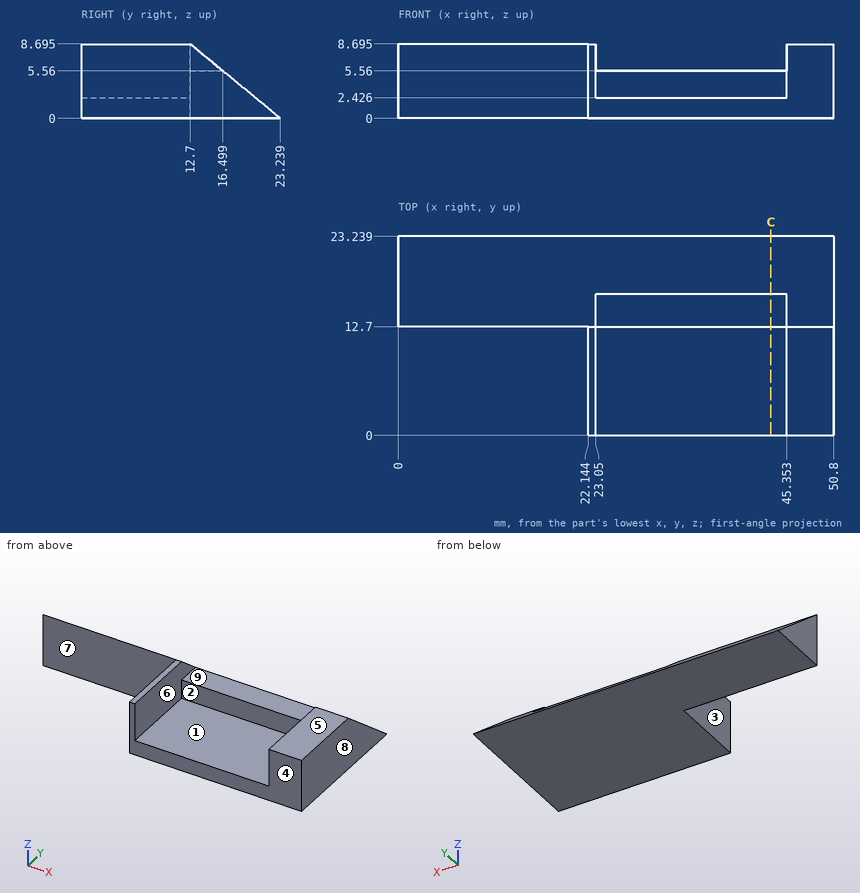
Verification items for this drawing (mm, ordinates from the low corner). A direction names the side the tool comes from. Coordinates: 2 decimals unless noted, no trailing zeros. Order: outer loops, then holes, each group sorted by start corner. A loop starts at its lowest first (then second) coordinate and runs counter-clockwise, first axis right, second up. Notation, with made-up numbers: (42, -38.75) -> (87, -38.75) arc R24 ccw to (87, -13.75) -> close; hole circle Ø4 at (80, 64). An arc over 180 degrees is marked (long way). Answer as CSV lines item,"result". Start each with the question number.
1) Release check for a two-part mould opening along X. For the marked faces 1, 2, 3 and 4 record: released by +X, released by -X, zero draft, split by the parting line, or undercut.
2) Gauge pin test, flat ends, axial feed: pin 1 Ø4 at (x, y) = (35.5, 6.5) entering from +Z; pin 2 Ø2.5 at (x, z) = (31.5, 4) entering from -Y; pin 3 Ø2.5 at (y, z) = (5.5, 4.5) entering from -X. Record the tip position at first contact, or that the pin passes through.
3) Material ranges on L1, parallel to Z at x = 35.5, y = 12.5; L2, parallel to X at y = 2.75, z = 0.5 (1 decimal); L3, parallel to Y at x = 11.5, z = 2.25, recorded low to high. Write a range as [from, to].
4) Set-up check for the marked faces 5, 6, 7, 8 and 9: record each of +Z, -Z, +X, -X, +Y, -Y from which the full face is reachable in a straight line by a thin tool's end or side.
5) Cross-section at C-C, the plane x = 43.5. Record the boundary of the cut face in (y, z).
Conclusion:
1,face 1,"undercut"
1,face 2,"undercut"
1,face 3,"released by -X"
1,face 4,"zero draft"
2,pin 1,"stops at z = 2.43"
2,pin 2,"stops at y = 12.7"
2,pin 3,"stops at x = 22.14"
3,L1,"z = [0, 2.43]"
3,L2,"x = [22.1, 50.8]"
3,L3,"y = [12.7, 20.51]"
4,face 5,"+Z, +X, -X, +Y, -Y"
4,face 6,"+Z, -Y"
4,face 7,"+Z, -Z, -X, -Y"
4,face 8,"+Z, -Z, +X, +Y, -Y"
4,face 9,"+Z, +Y, -Y"
5,outline,"(0, 0) -> (23.24, 0) -> (16.5, 5.56) -> (12.7, 5.56) -> (12.7, 2.43) -> (0, 2.43) -> close"
